Verification items for the finished model (mm, model axes). A direction names the side the tool comes from. Coordinates: 2 decimals unless noted, no trailing zeros. Order: outer loops, then holes, each group sorted by start corner. A loop starts at its lowest first (then second) coordinate and runs counter-clockwise, first axis right, second up. Notation, with made-up numbers: (68.25, 50) -> (109.25, 50) arc R9 cw to (109.25, 66) -> close; hole circle Ø2 at (16.5, 17). An arc over 180 degrees is marked (long way). Use CSV: the item, a comma, the result in double quotes. Start each with the question number.
1) Tool access check on faces 1 (the flat face through (0, 37, 17)), 2 (the flat face through (1.37, 19.59, 15.03)), 3 (the flat face through (-11, 10, 3.802)), 4 (the flat face through (10, 37, 0)). Record the directions out of +Z, -Z, +X, -X, +Y, -Y that give a thin tool (end or side, any length) a straight path to the whole face; none if there is none.
2) Sectioned sample at D-D on y = 13.5. Record the boundary of the cut face in (x, z) (3 decimals), then the cut area to 3 significant figures.
3) Release check for a two-part mould opening along Y. For faces 5 (the flat face through (-6.125, 58, -4)), 6 (the flat face through (1.405, 24.389, 15.028)), 7 (the flat face through (0.086, 55.645, 5.632)) record: released by +Y, released by -Y, zero draft, split by the parting line, or undercut.
4) Scan lines: line 1 along Y through (x, z) = (0, -15); line 2 along X through (y, z) = (43.75, 0) (3 decimals); line 3 along Y through (x, z) = (0, 11). Record each from-to range of solid material in increasing order.
5) Go/stop test with flat-tipped pins: pin 1 (2 mm diameter, centred on y = 39, z = -12.5, fed in from -X); pin 2 (1 mm diameter, centred on y = 22.5, z = 15, fed in from +X); pin 3 (1 mm diameter, centred on y = 47.5, z = 16, fed in from +X); pin 4 (3 mm diameter, centred on x = 6.5, z = -3.5, fed in from -Y). Record where each tip stops, or that it passes through.
6) Sectioned sample at B-B on y = 47. Give the number of separate pieces and of enclosed holes in the cut face, then the cut area to 3 significant figures.
7) Sectioned sample at A-A on y = 22. Record the boundary of the cut face in (x, z) (3 decimals), then the cut area to 3 significant figures.
from build123d import *

# Parameters (mm, degrees)
SKETCH1_R           = 18
SKETCH1_R_2         = 2
SKETCH1_W           = 10.25
SKETCH1_H           = 10.25
BOSS_EXTRUDE1_DEPTH = 57
CUT_EXTRUDE1_START  = -25
CUT_EXTRUDE1_DEPTH  = 25
SKETCH4_W           = 9.35
SKETCH4_H           = 9.35
CUT_EXTRUDE3_DEPTH  = 20.4
CUT_EXTRUDE4_START  = -40
CUT_EXTRUDE4_DEPTH  = 40
SKETCH6_R           = 1.5
CUT_EXTRUDE5_DEPTH  = 70.267597042
SKETCH7_R           = 3
CUT_EXTRUDE6_DEPTH  = 3
CUT_EXTRUDE7_DEPTH  = 4
CHAMFER1_SIZE       = 1
CHAMFER1_SIZE_2     = 2.747477419
CUT_EXTRUDE8_DEPTH  = 63.42595614
SKETCH12_R          = 1.4
CUT_EXTRUDE10_DEPTH = 20
SKETCH13_R          = 20
SKETCH13_R_2        = 1.4
BOSS_EXTRUDE2_DEPTH = 3
BOSS_EXTRUDE3_DEPTH = 3


with BuildPart() as part:
    # Sketch1 → Boss-Extrude1 (new body)
    with BuildSketch(Plane(origin=(0, 0, 0), x_dir=(1, 0, 0), z_dir=(0, 1, 0))):
        with Locations(Location((0, 0, 0), (0, 0, 90))):
            Circle(SKETCH1_R)
        with Locations(Location((-12, 0, 0), (0, 0, 90))):
            Circle(SKETCH1_R_2, mode=Mode.SUBTRACT)
        Rectangle(SKETCH1_W, SKETCH1_H, mode=Mode.SUBTRACT)
    extrude(amount=BOSS_EXTRUDE1_DEPTH)

    # Sketch2 → Cut-Extrude1 (cut)
    with BuildSketch(Plane(origin=(0, 57, 0), x_dir=(1, 0, 0), z_dir=(0, 1, 0)).offset(CUT_EXTRUDE1_START)):
        with BuildLine():
            Line((-10.8, 5), (-17.291616466, 5))
            ThreePointArc((-17.291616466, 5), (-18, 0), (-17.291616466, -5))
            Line((-17.291616466, -5), (-10.8, -5))
            ThreePointArc((-10.8, -5), (-5.8, 0), (-10.8, 5))
        make_face()
    extrude(amount=CUT_EXTRUDE1_DEPTH, mode=Mode.SUBTRACT)

    # Sketch4 → Cut-Extrude3 (cut)
    with BuildSketch(Plane(origin=(0, 0, 0), x_dir=(-1, 0, 0), z_dir=(0, -1, 0))):
        with Locations((11.135393506, 0.872889968)):
            Rectangle(SKETCH4_W, SKETCH4_H)
    extrude(amount=-CUT_EXTRUDE3_DEPTH, mode=Mode.SUBTRACT)

    # Sketch5 → Cut-Extrude4 (cut)
    with BuildSketch(Plane(origin=(0, 57, 0), x_dir=(1, 0, 0), z_dir=(0, 1, 0)).offset(CUT_EXTRUDE4_START)):
        with BuildLine():
            Line((5.916079783, 17), (-5.916079783, 17))
            ThreePointArc((-5.916079783, 17), (0, 18), (5.916079783, 17))
        make_face()
        with BuildLine():
            Line((5.916079783, -17), (-5.916079783, -17))
            ThreePointArc((-5.916079783, -17), (0, -18), (5.916079783, -17))
        make_face()
    extrude(amount=CUT_EXTRUDE4_DEPTH, mode=Mode.SUBTRACT)

    # Sketch6 → Cut-Extrude5 (cut, through all)
    with BuildSketch(Plane(origin=(0, 0, -17), x_dir=(-1, 0, 0), z_dir=(0, 0, -1))):
        with Locations((0, 47)):
            Circle(SKETCH6_R)
        with Locations((0, 22)):
            Circle(SKETCH6_R)
    extrude(amount=-CUT_EXTRUDE5_DEPTH, mode=Mode.SUBTRACT)

    # Sketch7 → Cut-Extrude6 (cut)
    with BuildSketch(Plane(origin=(0, 0, -17), x_dir=(-1, 0, 0), z_dir=(0, 0, -1))):
        with Locations((0, 47)):
            Circle(SKETCH7_R)
        with Locations((0, 22)):
            Circle(SKETCH7_R)
    extrude(amount=-CUT_EXTRUDE6_DEPTH, mode=Mode.SUBTRACT)

    # Sketch8 → Cut-Extrude7 (cut)
    with BuildSketch(Plane.XY.offset(17)):
        Polygon((0, 43.8), (2.771281292, 45.4), (2.771281292, 48.6), (0, 50.2), (-2.771281292, 48.6), (-2.771281292, 45.4), align=None)
        Polygon((0, 18.8), (2.771281292, 20.4), (2.771281292, 23.6), (0, 25.2), (-2.771281292, 23.6), (-2.771281292, 20.4), align=None)
    extrude(amount=-CUT_EXTRUDE7_DEPTH, mode=Mode.SUBTRACT)

    # Chamfer1
    # the kernel refuses this chamfer: 2.747477419, 1 mm, written as the material it takes off along each edge
    with BuildSketch(Plane(origin=(-5.125, 57, -5.125), x_dir=(0, 0.09904090225204956, -0.9950833631817488), z_dir=(1, 0, 0)), Plane(origin=(-5.125, 57, 5.125), x_dir=(-0.9950833631817488, 0.09904090225204956, 0), z_dir=(0, 0, -1)), Plane(origin=(5.125, 57, 5.125), x_dir=(0, 0.09904090225204956, 0.9950833631817488), z_dir=(-1, 0, 0)), Plane(origin=(5.125, 57, -5.125), x_dir=(0.9950833631817488, 0.09904090225204956, 0), z_dir=(0, 0, 1))) as chamfer1_piece_1:
        Polygon((CHAMFER1_SIZE * 0.995083363182, -CHAMFER1_SIZE * 0.099040902252), (-CHAMFER1_SIZE_2 * 0.0990409022684, -CHAMFER1_SIZE_2 * 0.995083363346), (0, 0), align=None)
    extrude(amount=10.25, mode=Mode.SUBTRACT)
    with BuildSketch(Plane(origin=(-5.125, 57, 5.125), x_dir=(-0.9950833631817488, 0.09904090225204956, 0), z_dir=(0, 0, -1))) as chamfer1_piece_2a_section:
        Polygon((CHAMFER1_SIZE * 0.995083363182, -CHAMFER1_SIZE * 0.099040902252), (-CHAMFER1_SIZE_2 * 0.0990409022684, -CHAMFER1_SIZE_2 * 0.995083363346), (0, 0), align=None)
    chamfer1_piece_2a = extrude(amount=17.377491449, mode=Mode.PRIVATE)
    chamfer1_piece_2a = split(chamfer1_piece_2a, bisect_by=Plane(origin=(-5.432505006, 56.059901151, -5.125), z_dir=(0, 0, -1)), keep=Keep.TOP, mode=Mode.PRIVATE)
    with BuildSketch(Plane(origin=(-12.252491449, 57, -5.125), x_dir=(0, 0.09904090225204956, -0.9950833631817488), z_dir=(1, 0, 0))) as chamfer1_piece_2b_section:
        Polygon((CHAMFER1_SIZE * 0.995083363182, -CHAMFER1_SIZE * 0.099040902252), (-CHAMFER1_SIZE_2 * 0.0990409022684, -CHAMFER1_SIZE_2 * 0.995083363346), (0, 0), align=None)
    chamfer1_piece_2b = extrude(amount=17.377491449, mode=Mode.PRIVATE)
    chamfer1_piece_2b = split(chamfer1_piece_2b, bisect_by=Plane(origin=(-5.125, 56.059901151, -5.432505006), z_dir=(-1, 0, 0)), keep=Keep.TOP, mode=Mode.PRIVATE)
    chamfer1_piece_2 = chamfer1_piece_2a & chamfer1_piece_2b
    add(chamfer1_piece_2, mode=Mode.SUBTRACT)
    with BuildSketch(Plane(origin=(5.125, 57, -12.252491449), x_dir=(0.9950833631817488, 0.09904090225204956, 0), z_dir=(0, 0, 1))) as chamfer1_piece_3a_section:
        Polygon((CHAMFER1_SIZE * 0.995083363182, -CHAMFER1_SIZE * 0.099040902252), (-CHAMFER1_SIZE_2 * 0.0990409022684, -CHAMFER1_SIZE_2 * 0.995083363346), (0, 0), align=None)
    chamfer1_piece_3a = extrude(amount=17.377491449, mode=Mode.PRIVATE)
    chamfer1_piece_3a = split(chamfer1_piece_3a, bisect_by=Plane(origin=(5.432505006, 56.059901151, -5.125), z_dir=(0, 0, -1)), keep=Keep.TOP, mode=Mode.PRIVATE)
    with BuildSketch(Plane(origin=(-5.125, 57, -5.125), x_dir=(0, 0.09904090225204956, -0.9950833631817488), z_dir=(1, 0, 0))) as chamfer1_piece_3b_section:
        Polygon((CHAMFER1_SIZE * 0.995083363182, -CHAMFER1_SIZE * 0.099040902252), (-CHAMFER1_SIZE_2 * 0.0990409022684, -CHAMFER1_SIZE_2 * 0.995083363346), (0, 0), align=None)
    chamfer1_piece_3b = extrude(amount=17.377491449, mode=Mode.PRIVATE)
    chamfer1_piece_3b = split(chamfer1_piece_3b, bisect_by=Plane(origin=(5.125, 56.059901151, -5.432505006), z_dir=(1, 0, 0)), keep=Keep.TOP, mode=Mode.PRIVATE)
    chamfer1_piece_3 = chamfer1_piece_3a & chamfer1_piece_3b
    add(chamfer1_piece_3, mode=Mode.SUBTRACT)
    with BuildSketch(Plane(origin=(5.125, 57, 5.125), x_dir=(0, 0.09904090225204956, 0.9950833631817488), z_dir=(-1, 0, 0))) as chamfer1_piece_4a_section:
        Polygon((CHAMFER1_SIZE * 0.995083363182, -CHAMFER1_SIZE * 0.099040902252), (-CHAMFER1_SIZE_2 * 0.0990409022684, -CHAMFER1_SIZE_2 * 0.995083363346), (0, 0), align=None)
    chamfer1_piece_4a = extrude(amount=17.377491449, mode=Mode.PRIVATE)
    chamfer1_piece_4a = split(chamfer1_piece_4a, bisect_by=Plane(origin=(-5.125, 56.059901151, 5.432505006), z_dir=(-1, 0, 0)), keep=Keep.TOP, mode=Mode.PRIVATE)
    with BuildSketch(Plane(origin=(-5.125, 57, 12.252491449), x_dir=(-0.9950833631817488, 0.09904090225204956, 0), z_dir=(0, 0, -1))) as chamfer1_piece_4b_section:
        Polygon((CHAMFER1_SIZE * 0.995083363182, -CHAMFER1_SIZE * 0.099040902252), (-CHAMFER1_SIZE_2 * 0.0990409022684, -CHAMFER1_SIZE_2 * 0.995083363346), (0, 0), align=None)
    chamfer1_piece_4b = extrude(amount=17.377491449, mode=Mode.PRIVATE)
    chamfer1_piece_4b = split(chamfer1_piece_4b, bisect_by=Plane(origin=(-5.432505006, 56.059901151, 5.125), z_dir=(0, 0, 1)), keep=Keep.TOP, mode=Mode.PRIVATE)
    chamfer1_piece_4 = chamfer1_piece_4a & chamfer1_piece_4b
    add(chamfer1_piece_4, mode=Mode.SUBTRACT)
    with BuildSketch(Plane(origin=(12.252491449, 57, 5.125), x_dir=(0, 0.09904090225204956, 0.9950833631817488), z_dir=(-1, 0, 0))) as chamfer1_piece_5a_section:
        Polygon((CHAMFER1_SIZE * 0.995083363182, -CHAMFER1_SIZE * 0.099040902252), (-CHAMFER1_SIZE_2 * 0.0990409022684, -CHAMFER1_SIZE_2 * 0.995083363346), (0, 0), align=None)
    chamfer1_piece_5a = extrude(amount=17.377491449, mode=Mode.PRIVATE)
    chamfer1_piece_5a = split(chamfer1_piece_5a, bisect_by=Plane(origin=(5.125, 56.059901151, 5.432505006), z_dir=(1, 0, 0)), keep=Keep.TOP, mode=Mode.PRIVATE)
    with BuildSketch(Plane(origin=(5.125, 57, -5.125), x_dir=(0.9950833631817488, 0.09904090225204956, 0), z_dir=(0, 0, 1))) as chamfer1_piece_5b_section:
        Polygon((CHAMFER1_SIZE * 0.995083363182, -CHAMFER1_SIZE * 0.099040902252), (-CHAMFER1_SIZE_2 * 0.0990409022684, -CHAMFER1_SIZE_2 * 0.995083363346), (0, 0), align=None)
    chamfer1_piece_5b = extrude(amount=17.377491449, mode=Mode.PRIVATE)
    chamfer1_piece_5b = split(chamfer1_piece_5b, bisect_by=Plane(origin=(5.432505006, 56.059901151, 5.125), z_dir=(0, 0, 1)), keep=Keep.TOP, mode=Mode.PRIVATE)
    chamfer1_piece_5 = chamfer1_piece_5a & chamfer1_piece_5b
    add(chamfer1_piece_5, mode=Mode.SUBTRACT)

    # Sketch9 → Cut-Extrude8 (cut, through all)
    with BuildSketch(Plane.XZ):
        with BuildLine():
            Line((-7.454203172, -7.297889968), (-15.454203172, -7.297889968))
            ThreePointArc((-15.454203172, -7.297889968), (-13.761984914, -9.955415688), (-11.632322635, -12.277178848))
            Line((-11.632322635, -12.277178848), (-7.454203172, -7.297889968))
        make_face()
    extrude(amount=-CUT_EXTRUDE8_DEPTH, mode=Mode.SUBTRACT)

    # Sketch12 → Cut-Extrude10 (cut)
    with BuildSketch(Plane(origin=(0, 57, 0), x_dir=(1, 0, 0), z_dir=(0, 1, 0))):
        with Locations(Location((10, 0, 0), (0, 0, 270))):
            Circle(SKETCH12_R)
        with Locations(Location((-9.192388155, -9.192388155, 0), (0, 0, 270))):
            Circle(SKETCH12_R)
    extrude(amount=-CUT_EXTRUDE10_DEPTH, mode=Mode.SUBTRACT)

    # Sketch13 → Boss-Extrude2 (add)
    with BuildSketch(Plane(origin=(0, 57, 0), x_dir=(1, 0, 0), z_dir=(0, 1, 0))):
        with Locations(Location((0, 0, 0), (0, 0, 270))):
            Circle(SKETCH13_R)
        with Locations(Location((10, 0, 0), (0, 0, 270))):
            Circle(SKETCH13_R_2, mode=Mode.SUBTRACT)
        with Locations(Location((-9.192388155, -9.192388155, 0), (0, 0, 270))):
            Circle(SKETCH13_R_2, mode=Mode.SUBTRACT)
        with BuildLine():
            Line((-10.8, 5), (-17.291616466, 5))
            Line((-17.291616466, 5), (-17.291616466, -5))
            Line((-17.291616466, -5), (-10.8, -5))
            ThreePointArc((-10.8, -5), (-7.959770503, -4.114984375), (-6.125, -1.773238563))
            Line((-6.125, -1.773238563), (-6.125, -6.125))
            Line((-6.125, -6.125), (6.125, -6.125))
            Line((6.125, -6.125), (6.125, 6.125))
            Line((6.125, 6.125), (-6.125, 6.125))
            Line((-6.125, 6.125), (-6.125, 1.773238563))
            ThreePointArc((-6.125, 1.773238563), (-7.959770503, 4.114984375), (-10.8, 5))
        make_face(mode=Mode.SUBTRACT)
        with BuildLine():
            Line((-7.454203172, 7.297889968), (-15.454203172, 7.297889968))
            ThreePointArc((-15.454203172, 7.297889968), (-13.761984914, 9.955415688), (-11.632322635, 12.277178848))
            Line((-11.632322635, 12.277178848), (-7.454203172, 7.297889968))
        make_face(mode=Mode.SUBTRACT)
    extrude(amount=BOSS_EXTRUDE2_DEPTH)

    # Sketch14 → Boss-Extrude3 (add)
    with BuildSketch(Plane(origin=(0, 60, 0), x_dir=(1, 0, 0), z_dir=(0, 1, 0))):
        with BuildLine():
            Line((12.855752194, 15.320888862), (14.321646009, 13.960317173))
            ThreePointArc((14.321646009, 13.960317173), (14.268984946, 15.373549926), (12.855752194, 15.320888862))
        make_face()
    extrude(amount=-BOSS_EXTRUDE3_DEPTH)


solid = part.part
Answers follow:
1,face 1,"+Z, +X, -X"
1,face 2,"+Z"
1,face 3,"-Y"
1,face 4,"+Y"
2,outline,"circle Ø36 at (0, 0); hole (-15.81, -5.548) -> (-6.46, -5.548) -> (-6.46, 3.802) -> (-15.81, 3.802) -> close; hole (-15.454, -7.298) arc R18 ccw to (-11.632, -12.277) -> (-7.454, -7.298) -> close; hole (-5.125, -5.125) -> (5.125, -5.125) -> (5.125, 5.125) -> (-5.125, 5.125) -> close"
2,area,"804 mm²"
3,face 5,"zero draft"
3,face 6,"undercut"
3,face 7,"released by +Y"
4,line 1,"y = 0 to 19, 25 to 44, 50 to 60"
4,line 2,"x = -5.8 to -5.125, 5.125 to 8.6, 11.4 to 18"
4,line 3,"y = 0 to 20.5, 23.5 to 45.5, 48.5 to 60"
5,pin 1,"stops at x = -13.85"
5,pin 2,"stops at x = 10.67"
5,pin 3,"stops at x = 9.15"
5,pin 4,"stops at y = 0"
6,separate pieces,"2"
6,enclosed holes,"3"
6,area,"664 mm²"
7,outline,"(-5.916, -17) -> (-3, -17) -> (-3, -14) -> (-1.5, -14) -> (-1.5, -5.125) -> (-5.125, -5.125) -> (-5.125, 5.125) -> (-1.5, 5.125) -> (-1.5, 13) -> (-2.771, 13) -> (-2.771, 17) -> (-5.916, 17) arc R18 ccw to start; (1.5, -14) -> (3, -14) -> (3, -17) -> (5.916, -17) arc R18 ccw to (5.916, 17) -> (2.771, 17) -> (2.771, 13) -> (1.5, 13) -> (1.5, 5.125) -> (5.125, 5.125) -> (5.125, -5.125) -> (1.5, -5.125) -> close; hole (-15.454, -7.298) arc R18 ccw to (-11.632, -12.277) -> (-7.454, -7.298) -> close; hole circle Ø4 at (-12, 0)"
7,area,"773 mm²"
